Source: CAD feature listing. Evaluate the final solid. Frame: model axes, mm. Face numbers are marked on the shaded views. A direction names the side the tool comes from. Give positions to 0.01 mm unless a question says otherwise; leave off trailing zeros. Write each loop counter-clockwise with the first axis right and the second up, starting at its lowest first coordinate (ties: lowest second). Pieces come first, ordered by that corner, then holes. Notation, with made-up numbers: (-15, 42) -> (44, 42) arc R36 ccw to (44, 80) -> close; hole circle Ø3 at (19, -14.75). An arc over 180 degrees is marked (long way). Use a Markdown table: item, result. Add a question column.
```python
from build123d import *

# Parameters (mm, degrees)
BOSS_EXTRUDE1_DEPTH = 19.05


with BuildPart() as part:
    # Sketch1 → Boss-Extrude1 (new body)
    with BuildSketch(Plane(origin=(0, 0, 0), x_dir=(1, 0, 0), z_dir=(0, 1, 0))):
        with BuildLine():
            Line((-31.75, 39.558423237), (-50.8, 39.558423237))
            Line((-50.8, 39.558423237), (-50.8, 20.508423237))
            Line((-50.8, 20.508423237), (-31.75, 20.508423237))
            ThreePointArc((-31.75, 20.508423237), (-28.575, 17.333423237), (-31.75, 14.158423237))
            Line((-31.75, 14.158423237), (-31.75, -4.891576763))
            ThreePointArc((-31.75, -4.891576763), (-28.575, -8.066576763), (-31.75, -11.241576763))
            Line((-31.75, -11.241576763), (-50.8, -11.241576763))
            Line((-50.8, -11.241576763), (-50.8, -30.291576763))
            Line((-50.8, -30.291576763), (-31.75, -30.291576763))
            ThreePointArc((-31.75, -30.291576763), (-28.575, -33.466576763), (-31.75, -36.641576763))
            Line((-31.75, -36.641576763), (-31.75, -62.041576763))
            Line((-31.75, -62.041576763), (-6.35, -62.041576763))
            ThreePointArc((-6.35, -62.041576763), (-3.175, -58.866576763), (0, -62.041576763))
            Line((0, -62.041576763), (0, -79.821576763))
            Line((0, -79.821576763), (17.78, -79.821576763))
            Line((17.78, -79.821576763), (17.78, -62.041576763))
            ThreePointArc((17.78, -62.041576763), (20.955, -58.866576763), (24.13, -62.041576763))
            Line((24.13, -62.041576763), (43.18, -62.041576763))
            ThreePointArc((43.18, -62.041576763), (46.355, -58.866576763), (49.53, -62.041576763))
            Line((49.53, -62.041576763), (49.53, -79.821576763))
            Line((49.53, -79.821576763), (67.31, -79.821576763))
            Line((67.31, -79.821576763), (67.31, -62.041576763))
            ThreePointArc((67.31, -62.041576763), (70.485, -58.866576763), (73.66, -62.041576763))
            Line((73.66, -62.041576763), (106.027076755, -62.041576763))
            Line((106.027076755, -62.041576763), (106.027076755, 71.308423237))
            Line((106.027076755, 71.308423237), (78.74, 71.308423237))
            ThreePointArc((78.74, 71.308423237), (75.565, 68.133423237), (72.39, 71.308423237))
            Line((72.39, 71.308423237), (72.39, 91.628423237))
            Line((72.39, 91.628423237), (52.07, 91.628423237))
            Line((52.07, 91.628423237), (52.07, 71.308423237))
            ThreePointArc((52.07, 71.308423237), (48.895, 68.133423237), (45.72, 71.308423237))
            Line((45.72, 71.308423237), (26.67, 71.308423237))
            ThreePointArc((26.67, 71.308423237), (23.495, 68.133423237), (20.32, 71.308423237))
            Line((20.32, 71.308423237), (20.32, 91.628423237))
            Line((20.32, 91.628423237), (0, 91.628423237))
            Line((0, 91.628423237), (0, 71.308423237))
            ThreePointArc((0, 71.308423237), (-3.175, 68.133423237), (-6.35, 71.308423237))
            Line((-6.35, 71.308423237), (-31.75, 71.308423237))
            Line((-31.75, 71.308423237), (-31.75, 45.908423237))
            ThreePointArc((-31.75, 45.908423237), (-28.575, 42.733423237), (-31.75, 39.558423237))
        make_face()
    extrude(amount=BOSS_EXTRUDE1_DEPTH)


solid = part.part
```
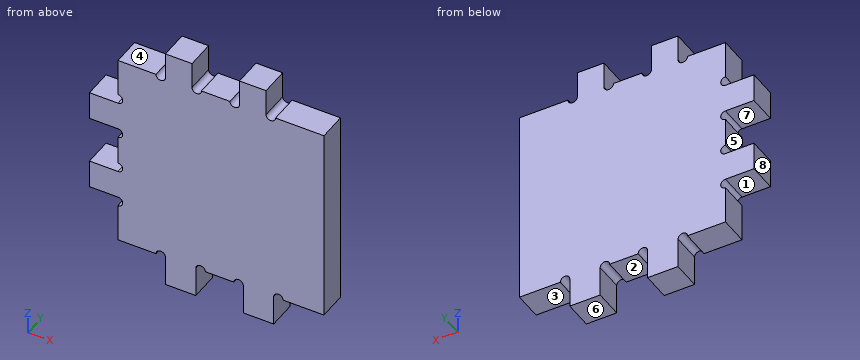
(1) Access query for the marked faces 1, 2, 3, 4 and 5. Directions: +Z, -Z, +X, -X, +Y, -Y. A direction counts if a zero-diameter tool reaches every point of the face in a straight line with its end or side. Return the directions, or none.
(2) First-contact query: pin 1 Ø5 at (x, y) = (-16, 8.5) entering from -Z; pin 2 Ø9.5 at (x, y) = (33.5, 14.5) entering from +Z; pin 3 Ø9 at (y, z) = (8, 74.5) entering from +X. Flat tips, straight axial feed; report the tip coordinate or a pass-through.
(3) Mould query, pull axis Z, two halves, no side actions, for the marked faces 6, 7 and 8. Classes: +Z half, -Z half, draft (parallel to the pull), parting line (faces both ways), or undercut.
(4) Material intervals for L1, parallel to X at y = 8.25, z = -76.5; L2, parallel to Z at x = -43.5, y = 14.25; L3, parallel to Z at x = 98.5, y = 9.25, sorted ascending.
(5) Cut plane B-B on z = -64.5. Return the cut outline in (x, y), then the cut area to 3 significant figures.
(6) Cut plane A-A on x = 82.5. Return the cut outline in (y, z), then the cut area to 3 significant figures.
Output:
| question | item | result |
|---|---|---|
| 1 | face 1 | -Z, -X, +Y, -Y |
| 1 | face 2 | -Z, +Y, -Y |
| 1 | face 3 | -Z, +X, +Y, -Y |
| 1 | face 4 | +Z, -X, +Y, -Y |
| 1 | face 5 | -X, +Y, -Y |
| 2 | pin 1 | z = -71.31 |
| 2 | pin 2 | z = 62.04 |
| 2 | pin 3 | x = 67.31 |
| 3 | face 6 | -Z half |
| 3 | face 7 | undercut |
| 3 | face 8 | draft |
| 4 | L1 | 0 to 20.32, 52.07 to 72.39 |
| 4 | L2 | -39.56 to -20.51, 11.24 to 30.29 |
| 4 | L3 | -71.31 to 62.04 |
| 5 | outline | (-31.75, 0) -> (106.03, 0) -> (106.03, 19.05) -> (-31.75, 19.05) -> close |
| 5 | area | 2,620 mm^2 |
| 6 | outline | (0, -71.31) -> (19.05, -71.31) -> (19.05, 62.04) -> (0, 62.04) -> close |
| 6 | area | 2,540 mm^2 |
